Work out the finished part from the listing and answer in its coordinate system (mm). A direction names the side the tool comes from. Coordinates: 2 decimals unless noted, no trailing zeros. Write each loop counter-clockwise with the first axis right and the second up, starting at its lowest first coordinate (ties: lowest second). Pieces come first, ordered by that corner, then holes. Notation, with made-up numbers: M 60,-17.75 L 101,-17.75 A28 ccw 101,11.25 Z; hole C -3,21.25 d2. An arc over 180 degrees is marked long. Use CSV: the item, a comma, the result in double quotes.
from build123d import *

# Parameters (mm, degrees)
TAP_DRILL_FOR_M4_TAP1_D     = 3.3
TAP_DRILL_FOR_M4_TAP1_DEPTH = 10
TAP_DRILL_FOR_M4_TAP1_TIP   = 0.991420021
CHAMFER1_SIZE               = 0.25
SKETCH4_W                   = 3
SKETCH4_H                   = 3
CUT_EXTRUDE1_DEPTH          = 25
FILLET1_R                   = 1.5


with BuildPart() as part:
    # Sketch1 → Revolve1 (revolve)
    with BuildSketch(Plane.XY, mode=Mode.PRIVATE) as revolve1_sk:
        Polygon((0, 55.365578046), (5, 55.365578046), (5, 40.865578046), (8.5, 40.865578046), (8.5, 38.865578046), (7.5, 38.865578046), (7.5, 31.065578046), (5, 31.065578046), (5, 5.565578046), (0, 5.565578046), align=None)
    revolve(revolve1_sk.sketch.rotate(Axis((0, 0, 0), (0, 1, 0)), 90), axis=Axis((0, 0, 0), (0, 1, 0)))

    # Tap Drill for M4 Tap1
    with Locations(Plane(origin=(0, 5.565578046, 0), x_dir=(-1, 0, 0), z_dir=(0, -1, 0))):
        with Locations((0, 0)):
            Hole(TAP_DRILL_FOR_M4_TAP1_D / 2, depth=TAP_DRILL_FOR_M4_TAP1_DEPTH)
            with Locations((0, 0, -(TAP_DRILL_FOR_M4_TAP1_DEPTH + TAP_DRILL_FOR_M4_TAP1_TIP / 2))):  # 118° drill point
                Cone(0, TAP_DRILL_FOR_M4_TAP1_D / 2, TAP_DRILL_FOR_M4_TAP1_TIP, mode=Mode.SUBTRACT)

    # Chamfer1
    chamfer1_edges = [part.edges().sort_by_distance(p)[0] for p in [
        (0, 55.365578046, 5),
        (-1.65, 5.565578046, 0),
        (0, 5.565578046, 5),
        (0, 31.065578046, 7.5),
        (0, 38.865578046, 8.5),
        (0, 40.865578046, 8.5),
    ]]
    chamfer(chamfer1_edges, length=CHAMFER1_SIZE)

    # Sketch4 → Cut-Extrude1 (cut)
    with BuildSketch(Plane.XZ.offset(-5.565578046)):
        with Locations((0, 4.65)):
            Rectangle(SKETCH4_W, SKETCH4_H)
    extrude(amount=-CUT_EXTRUDE1_DEPTH, mode=Mode.SUBTRACT)

    # Fillet1
    fillet1_edges = [part.edges().sort_by_distance(p)[0] for p in [
        (1.5, 30.565578046, 3.959848004),
        (-1.5, 30.565578046, 3.959848004),
    ]]
    fillet(fillet1_edges, radius=FILLET1_R - 0.0001)  # a hair under: the kernel refuses the full size


solid = part.part
Item 1: A tool of negligible diameter and unlimited length cuts with its end or side. For faces 1 (the face through (0, 48, 5)), 2 (the face through (1.072, 30.115, 4.088)), 3 (the face through (-1.5, 18.26, -4.77)), from which of +Z, -Z, +X, -X, +Y, -Y can it reach the whole face along a straight path? Write none if from no direction.
Answer:
face 1,"+Y"
face 2,"+Z, -Y"
face 3,"-Y"
Item 2: Given pin 1 (1.8 mm diameter, centred on y = 18.5, z = 4.5, fed in from -X); pin 2 (3 mm diameter, centred on x = 5.5, y = 30, fed in from -Z); pin 3 (6 mm diameter, centred on y = 48, z = 1, fed in from +X); pin 4 (1 mm diameter, centred on x = 6, y = 19, fed in from -Z), each flat-ended and moving along its own axis, determine where each tip first touches the part or whether it passes through.
Answer:
pin 1,"stops at x = -3.47"
pin 2,"stops at z = -5.78"
pin 3,"stops at x = 5"
pin 4,"passes through"
Item 3: The part is cut by section B-B (y = 19). Write down the section's boundary in (x, z).
Answer:
outline,"M -1.5,3.15 L -1.5,4.77 A5 ccw long 1.5,4.77 L 1.5,3.15 Z"
Item 4: The part is cut by section A-A (y = 51). Write down the section's boundary in (x, z).
Answer:
outline,"C 0,0 d10"
Item 5: Consider probe 1 along X at (y, z) = (8.5, 0); probe 2 along Z at (x, y) = (-0.25, 25); probe 3 along Y at (x, z) = (-0.25, -4.75). Determine where each line is inside the solid, lowest interval first.
Answer:
probe 1,"x = -5 to -1.65, 1.65 to 5"
probe 2,"z = -4.99 to 3.15"
probe 3,"y = 5.57 to 55.36"
Item 6: For a pull along X with two mould halves and no side action, classify faces 4 (the face through (7, 38.866, -4)), 5 (the face through (0.062, 16.385, 0.28)), 6 (the face through (-6.324, 35.038, -4.032)), 7 (the face through (-1.049, 30.138, 4.088)) as released by +X, released by -X, zero draft, split by the parting line, or undercut.
Answer:
face 4,"zero draft"
face 5,"undercut"
face 6,"split by the parting line"
face 7,"undercut"
